Could you check a few things on this model? Use its own coordinates, in mm. A direction names the side the tool comes from. Round coordinates to 2 decimals unless told otherwise and drop trailing zeros. Loops run counter-clockwise (first coordinate to the right, second up) from the corner with the lowest first, then second, coordinate; pieces in that order, holes last. Notation, with made-up numbers: M 85.25,61.5 L 97.25,61.5 A14 cw 97.25,74.5 Z; hole C 22.5,-0.75 d5. An arc over 180 degrees is marked long. Return JSON: item names as keys, results as strings. Group by question number.
```python
from build123d import *

# Parameters (mm, degrees)
F0_W     = 25
F0_H     = 25
F1_DEPTH = 762
F3_DEPTH = 12.5
F4_W     = 22
F4_H     = 22
F5_DEPTH = 762.001


with BuildPart() as f1:
    # F0 (on Right) → F1 (new body)
    with BuildSketch(Plane.YZ):
        Rectangle(F0_W, F0_H)
    extrude(amount=F1_DEPTH)

    # F2 (on Front) → F3 (cut, symmetric)
    with BuildSketch(Plane.XZ):
        Polygon((35.352029, -22.745401), (0, 12.606628), (0, -26.686775), align=None)
        Polygon((762, -22.745401), (762, 12.5), (732.63703, -16.86297), align=None)
    extrude(amount=F3_DEPTH, both=True, mode=Mode.SUBTRACT)

    # F4 (on Right) → F5 (cut, through all)
    with BuildSketch(Plane.YZ):
        Rectangle(F4_W, F4_H)
    extrude(amount=F5_DEPTH, mode=Mode.SUBTRACT)


solid = f1.part
```
1. If we section it at C-C, the plane z = 2.5: Please give me the cut outline in (x, y), then the cut area to 3 significant figures.
2. On a 3-axis mill with a long thin cutter (end or side, diameter ignored), from which of +Z, -Z, +X, -X, +Y, -Y can I reach the whole of each face in a straight line? I mean faces 4 (the face through (12.665, 11.169, -0.058)), 5 (the face through (376, 0, 11)). Say none if no direction works.
3. We'd pull the mould along Z, two halves only. Please class faces 1 (the face through (749.6, -11.2, 0.1)), 2 (the face through (376, 11, 0)), 3 (the face through (376, 12.5, 0)): +Z half, -Z half, draft (parallel to the pull), parting line (faces both ways), or undercut.
4. I need wall thicknesses on probe 1 along Z at (x, y) = (651, 7.75). Which ranges of the line are inside material? Lowest first, please.
5. If we section it at B-B, the plane x = 319.5: Please give me the cut outline in (y, z).
6. If we section it at A-A, the plane y = 6.25: Please give me the cut outline in (x, z).
Geometry results:
{
 "1": {"outline": "M 10.11,-12.5 L 752,-12.5 L 752,-11 L 10.11,-11 Z; M 10.11,11 L 752,11 L 752,12.5 L 10.11,12.5 Z", "area": "2,230 mm^2"},
 "2": {"face 4": "-Z, -X, +Y, -Y", "face 5": "+X, -X"},
 "3": {"face 1": "-Z half", "face 2": "undercut", "face 3": "draft"},
 "4": {"probe 1": "-12.5 to -11, 11 to 12.5"},
 "5": {"outline": "M -12.5,-12.5 L 12.5,-12.5 L 12.5,12.5 L -12.5,12.5 Z; hole M -11,-11 L 11,-11 L 11,11 L -11,11 Z"},
 "6": {"outline": "M 0.11,12.5 L 1.61,11 L 760.5,11 L 762,12.5 Z; M 23.61,-11 L 25.11,-12.5 L 737,-12.5 L 738.5,-11 Z"}
}
